Model file for the job. Use its own axes, mm. Face numbers are marked on the shaded views. A direction names the side the tool comes from. Coordinates: 2 decimals unless noted, no trailing zeros. Write each loop counter-clockwise with the first axis right and the second up, starting at its lowest first coordinate (ties: lowest second). Pieces come first, ordered by that corner, then holes.
Q1. Drill centre lines: probe 1 along Z at (x, y) = (-2, 1); probe 2 along X at (y, z) = (1.5, 11.5); probe 3 along Y at (x, z) = (-1.4, 6). Where is each one in solid material? Low to high.
Q2. Which spindle directions (+Z, -Z, +X, -X, +Y, -Y) get a long thin tool onto all of the face, cutting with end or side? Do the marked faces 1 and 2. Say none if no direction does.
Q3. Band-saw the part on A-A, the plane x = 0. Write the cut outline in (y, z), plus the area to 3 significant figures.
Q4. Band-saw the part on B-B, the plane z = 26. Write the cut outline in (x, y), plus the area to 3 significant figures.
Q5. Pin check, flat tip, straight feed: P1, Ø1.5, axis at x = -0.5, y = -1.5, coming from the +Z side. Stop position of the tip, or through.
Q6. Band-saw the part on C-C, the plane y = 1.95. Write the cut outline in (x, z).
from build123d import *

# Parameters (mm, degrees)
EXTRUDE_1_DEPTH = 40
SKETCH_2_R      = 1.5
EXTRUDE_2_DEPTH = 5
FILLET_1_R      = 1.5


with BuildPart() as part:
    # 草图1 → 凸台-拉伸1 (new body)
    with BuildSketch(Plane.XY):
        Polygon((2.690452254, 0), (1.345226127, 2.33), (-1.345226127, 2.33), (-2.690452254, 0), (-1.345226127, -2.33), (1.345226127, -2.33), align=None)
    extrude(amount=EXTRUDE_1_DEPTH)

    # 草图2 → 凸台-拉伸2 (add)
    with BuildSketch(Plane.XY.offset(40)):
        Circle(SKETCH_2_R)
    extrude(amount=EXTRUDE_2_DEPTH)

    # 圆角1
    fillet_1_edges = [part.edges().sort_by_distance(p)[0] for p in [
        (-1.5, 0, 45),
    ]]
    fillet(fillet_1_edges, radius=FILLET_1_R)


solid = part.part
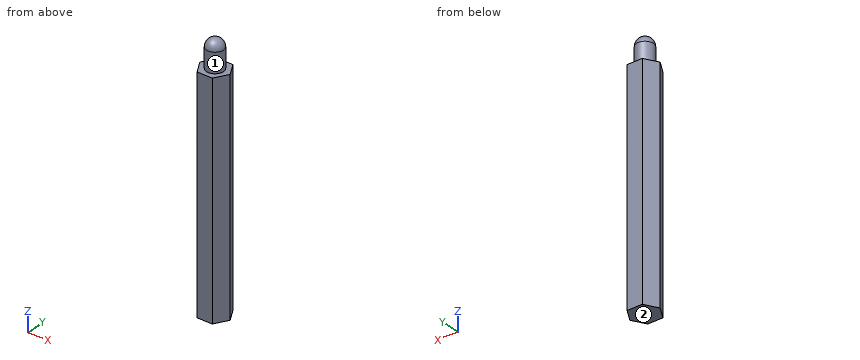
Answer sheet:
1. probe 1: z = 0 to 40
1. probe 2: x = -1.82 to 1.82
1. probe 3: y = -2.24 to 2.24
2. face 1: +Z
2. face 2: -Z, +X, -X, +Y, -Y
3. outline: (-2.33, 0) - (2.33, 0) - (2.33, 40) - (1.5, 40) - (1.5, 43.5) arc R1.5 ccw to (-1.5, 43.5) - (-1.5, 40) - (-2.33, 40) - close
3. area: 200 mm2
4. outline: (-2.69, 0) - (-1.35, -2.33) - (1.35, -2.33) - (2.69, 0) - (1.35, 2.33) - (-1.35, 2.33) - close
4. area: 18.8 mm2
5. P1: stops at z = 44.75
6. outline: (-1.56, 0) - (1.56, 0) - (1.56, 40) - (-1.56, 40) - close
